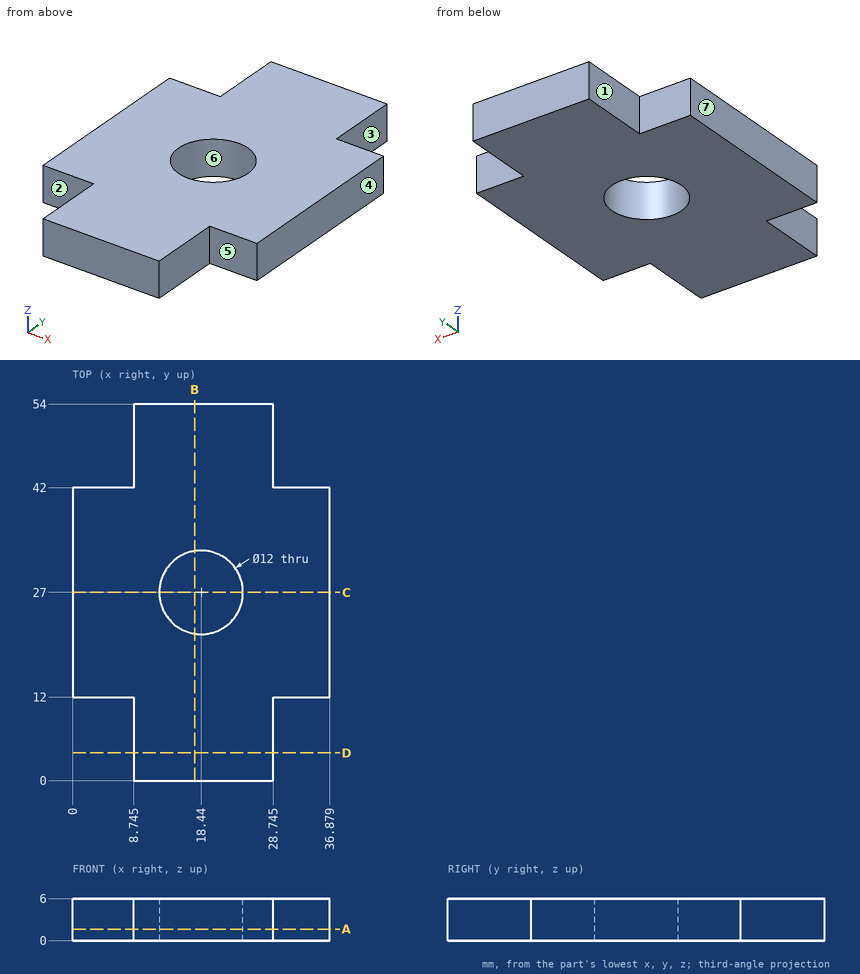
Verification items for this drawing (mm, ordinates from the low corner). A direction names the side the tool comes from. Coordinates: 2 decimals unless noted, no trailing zeros. Order: outer loops, then holes, each group sorted by start corner. A loop starts at its lowest first (then second) coordinate and runs counter-clockwise, first axis right, second up. Notation, with made-up numbers: (49, -37) - (95, -37) arc R34 cw to (95, -6) - close; hole circle Ø3 at (13, -23.75). An arc over 180 degrees is marked (long way). Answer as a JSON object with one key per item and string values. Group by question number.
Item 1: Tool access check on the marked faces 1, 2 and 3. Record the directions out of +Z, -Z, +X, -X, +Y, -Y that give a thin tool (end or side, any length) a straight path to the whole face; none if there is none.
Item 2: Draft check along X on the marked faces 4, 5, 6 and 7. Enter one of: +X half, -X half, draft (parallel to the pull), parting line (faces both ways), or undercut.
Item 3: Sectioned sample at D-D, the plane y = 4. Record the cut outline in (x, z) (1 decimal).
Item 4: Depth check by flat-ended pin: pin 1 Ø3 at (y, z) = (5, 3.5) entering from +X (3 decimals); pin 2 Ø3 at (x, z) = (32, 2.5) entering from +Y; pin 3 Ø10 at (x, y) = (28.5, 15) entering from -Z; pin 4 Ø3 at (x, z) = (5.5, 1.5) entering from -Y. Enter the tip coordinate at first touch or a pass-through.
Item 5: Scan lines: probe 1 along Y at (x, z) = (18.5, 1.4); probe 2 along X at (y, z) = (52, 0.6) (1 decimal); probe 3 along Y at (x, z) = (31.5, 3.85). Record each from-to range of solid material in increasing order.
Item 6: Sectioned sample at B-B, the plane x = 17.5. Record the cut outline in (y, z), and give its area (3 significant figures).
Item 7: Sectioned sample at C-C, the plane y = 27. Record the cut outline in (x, z).
Item 8: Sectioned sample at A-A, the plane z = 1.65. Record the cut outline in (x, y) (1 decimal), and give its area (3 significant figures).
Resolved:
{
 "1": {"face 1": "+Z, -Z, -X, +Y", "face 2": "+Z, -Z, -X, -Y", "face 3": "+Z, -Z, +X, +Y"},
 "2": {"face 4": "+X half", "face 5": "draft", "face 6": "undercut", "face 7": "-X half"},
 "3": {"outline": "(8.7, 0) - (28.7, 0) - (28.7, 6) - (8.7, 6) - close"},
 "4": {"pin 1": "x = 28.745", "pin 2": "y = 42", "pin 3": "z = 0", "pin 4": "y = 12"},
 "5": {"probe 1": "0 to 21, 33 to 54", "probe 2": "8.7 to 28.7", "probe 3": "12 to 42"},
 "6": {"outline": "(0, 0) - (21.07, 0) - (21.07, 6) - (0, 6) - close; (32.93, 0) - (54, 0) - (54, 6) - (32.93, 6) - close", "area": "253 mm^2"},
 "7": {"outline": "(0, 0) - (12.44, 0) - (12.44, 6) - (0, 6) - close; (24.44, 0) - (36.88, 0) - (36.88, 6) - (24.44, 6) - close"},
 "8": {"outline": "(0, 12) - (8.7, 12) - (8.7, 0) - (28.7, 0) - (28.7, 12) - (36.9, 12) - (36.9, 42) - (28.7, 42) - (28.7, 54) - (8.7, 54) - (8.7, 42) - (0, 42) - close; hole circle Ø12 at (18.4, 27)", "area": "1,470 mm^2"}
}
